from build123d import *

# Parameters (mm, degrees)
PLENUM_START          = -375
PLENUM_DEPTH          = 415
PLENUM_START_2        = -360
PLENUM_RIBS_DEPTH     = 385
RUNNER_START          = -6.1
RUNNER_1_DEPTH        = 36
RUNNER_START_2        = -29.9
RUNNER_2_DEPTH        = 36
RUNNER_START_3        = -117.86
RUNNER_3_DEPTH        = 36
RUNNER_START_4        = -141.66
RUNNER_4_DEPTH        = 36
RUNNER_START_5        = -229.62
RUNNER_5_DEPTH        = 36
RUNNER_START_6        = -253.42
RUNNER_6_DEPTH        = 36
RUNNER_START_7        = -341.38
RUNNER_7_DEPTH        = 36
RUNNER_START_8        = -365.18
RUNNER_8_DEPTH        = 36
THROTTLE_START        = 40
SKETCH11_R            = 44
THROTTLE_FLANGE_DEPTH = 8
THROTTLE_START_2      = 48
SKETCH12_R            = 36
THROTTLE_BODY_DEPTH   = 40
THROTTLE_START_3      = 50
SKETCH13_R            = 29
THROTTLE_BORE_DEPTH   = 40
FUEL_START            = -360
SKETCH14_R            = 8
FUEL_RAILS_DEPTH      = 390


with BuildPart() as part:
    # Sketch1 → Plenum (new body)
    with BuildSketch(Plane.XY.offset(PLENUM_START)):
        with BuildLine():
            Line((-50, 285), (50, 285))
            ThreePointArc((50, 285), (64.142135624, 290.857864376), (70, 305))
            Line((70, 305), (70, 335))
            ThreePointArc((70, 335), (64.142135624, 349.142135624), (50, 355))
            Line((50, 355), (-50, 355))
            ThreePointArc((-50, 355), (-64.142135624, 349.142135624), (-70, 335))
            Line((-70, 335), (-70, 305))
            ThreePointArc((-70, 305), (-64.142135624, 290.857864376), (-50, 285))
        make_face()
    extrude(amount=PLENUM_DEPTH)

    # Sketch2 → Plenum Ribs (add)
    with BuildSketch(Plane.XY.offset(PLENUM_START_2)):
        with BuildLine():
            Line((-50, 350), (-42, 350))
            Line((-42, 350), (-42, 359))
            ThreePointArc((-42, 359), (-42.878679656, 361.121320344), (-45, 362))
            Line((-45, 362), (-47, 362))
            ThreePointArc((-47, 362), (-49.121320344, 361.121320344), (-50, 359))
            Line((-50, 359), (-50, 350))
        make_face()
        with BuildLine():
            Line((-4, 350), (4, 350))
            Line((4, 350), (4, 359))
            ThreePointArc((4, 359), (3.121320344, 361.121320344), (1, 362))
            Line((1, 362), (-1, 362))
            ThreePointArc((-1, 362), (-3.121320344, 361.121320344), (-4, 359))
            Line((-4, 359), (-4, 350))
        make_face()
        with BuildLine():
            Line((42, 350), (50, 350))
            Line((50, 350), (50, 359))
            ThreePointArc((50, 359), (49.121320344, 361.121320344), (47, 362))
            Line((47, 362), (45, 362))
            ThreePointArc((45, 362), (42.878679656, 361.121320344), (42, 359))
            Line((42, 359), (42, 350))
        make_face()
    extrude(amount=PLENUM_RIBS_DEPTH)

    # Sketch3 → Runner 1 (add)
    with BuildSketch(Plane.XY.offset(RUNNER_START)):
        with BuildLine():
            Line((132.900719524, 234.724096015), (115.737566336, 251.887249203))
            ThreePointArc((115.737566336, 251.887249203), (114.502776925, 252.936394099), (113.114761283, 253.772350127))
            Line((113.114761283, 253.772350127), (28.879343102, 295.60957816))
            Line((28.879343102, 295.60957816), (51.120656898, 340.39042184))
            Line((51.120656898, 340.39042184), (142.684314275, 294.913475254))
            ThreePointArc((142.684314275, 294.913475254), (144.072329917, 294.077519226), (145.307119327, 293.02837433))
            Line((145.307119327, 293.02837433), (168.256058583, 270.079435074))
            Line((168.256058583, 270.079435074), (132.900719524, 234.724096015))
        make_face()
    extrude(amount=RUNNER_1_DEPTH)

    # Sketch4 → Runner 2 (add)
    with BuildSketch(Plane.XY.offset(RUNNER_START_2)):
        with BuildLine():
            Line((-168.256058583, 270.079435074), (-145.307119327, 293.02837433))
            ThreePointArc((-145.307119327, 293.02837433), (-144.072329917, 294.077519226), (-142.684314275, 294.913475254))
            Line((-142.684314275, 294.913475254), (-51.120656898, 340.39042184))
            Line((-51.120656898, 340.39042184), (-28.879343102, 295.60957816))
            Line((-28.879343102, 295.60957816), (-113.114761283, 253.772350127))
            ThreePointArc((-113.114761283, 253.772350127), (-114.502776925, 252.936394099), (-115.737566336, 251.887249203))
            Line((-115.737566336, 251.887249203), (-132.900719524, 234.724096015))
            Line((-132.900719524, 234.724096015), (-168.256058583, 270.079435074))
        make_face()
    extrude(amount=RUNNER_2_DEPTH)

    # Sketch5 → Runner 3 (add)
    with BuildSketch(Plane.XY.offset(RUNNER_START_3)):
        with BuildLine():
            Line((132.900719524, 234.724096015), (115.737566336, 251.887249203))
            ThreePointArc((115.737566336, 251.887249203), (114.502776925, 252.936394099), (113.114761283, 253.772350127))
            Line((113.114761283, 253.772350127), (28.879343102, 295.60957816))
            Line((28.879343102, 295.60957816), (51.120656898, 340.39042184))
            Line((51.120656898, 340.39042184), (142.684314275, 294.913475254))
            ThreePointArc((142.684314275, 294.913475254), (144.072329917, 294.077519226), (145.307119327, 293.02837433))
            Line((145.307119327, 293.02837433), (168.256058583, 270.079435074))
            Line((168.256058583, 270.079435074), (132.900719524, 234.724096015))
        make_face()
    extrude(amount=RUNNER_3_DEPTH)

    # Sketch6 → Runner 4 (add)
    with BuildSketch(Plane.XY.offset(RUNNER_START_4)):
        with BuildLine():
            Line((-168.256058583, 270.079435074), (-145.307119327, 293.02837433))
            ThreePointArc((-145.307119327, 293.02837433), (-144.072329917, 294.077519226), (-142.684314275, 294.913475254))
            Line((-142.684314275, 294.913475254), (-51.120656898, 340.39042184))
            Line((-51.120656898, 340.39042184), (-28.879343102, 295.60957816))
            Line((-28.879343102, 295.60957816), (-113.114761283, 253.772350127))
            ThreePointArc((-113.114761283, 253.772350127), (-114.502776925, 252.936394099), (-115.737566336, 251.887249203))
            Line((-115.737566336, 251.887249203), (-132.900719524, 234.724096015))
            Line((-132.900719524, 234.724096015), (-168.256058583, 270.079435074))
        make_face()
    extrude(amount=RUNNER_4_DEPTH)

    # Sketch7 → Runner 5 (add)
    with BuildSketch(Plane.XY.offset(RUNNER_START_5)):
        with BuildLine():
            Line((132.900719524, 234.724096015), (115.737566336, 251.887249203))
            ThreePointArc((115.737566336, 251.887249203), (114.502776925, 252.936394099), (113.114761283, 253.772350127))
            Line((113.114761283, 253.772350127), (28.879343102, 295.60957816))
            Line((28.879343102, 295.60957816), (51.120656898, 340.39042184))
            Line((51.120656898, 340.39042184), (142.684314275, 294.913475254))
            ThreePointArc((142.684314275, 294.913475254), (144.072329917, 294.077519226), (145.307119327, 293.02837433))
            Line((145.307119327, 293.02837433), (168.256058583, 270.079435074))
            Line((168.256058583, 270.079435074), (132.900719524, 234.724096015))
        make_face()
    extrude(amount=RUNNER_5_DEPTH)

    # Sketch8 → Runner 6 (add)
    with BuildSketch(Plane.XY.offset(RUNNER_START_6)):
        with BuildLine():
            Line((-168.256058583, 270.079435074), (-145.307119327, 293.02837433))
            ThreePointArc((-145.307119327, 293.02837433), (-144.072329917, 294.077519226), (-142.684314275, 294.913475254))
            Line((-142.684314275, 294.913475254), (-51.120656898, 340.39042184))
            Line((-51.120656898, 340.39042184), (-28.879343102, 295.60957816))
            Line((-28.879343102, 295.60957816), (-113.114761283, 253.772350127))
            ThreePointArc((-113.114761283, 253.772350127), (-114.502776925, 252.936394099), (-115.737566336, 251.887249203))
            Line((-115.737566336, 251.887249203), (-132.900719524, 234.724096015))
            Line((-132.900719524, 234.724096015), (-168.256058583, 270.079435074))
        make_face()
    extrude(amount=RUNNER_6_DEPTH)

    # Sketch9 → Runner 7 (add)
    with BuildSketch(Plane.XY.offset(RUNNER_START_7)):
        with BuildLine():
            Line((132.900719524, 234.724096015), (115.737566336, 251.887249203))
            ThreePointArc((115.737566336, 251.887249203), (114.502776925, 252.936394099), (113.114761283, 253.772350127))
            Line((113.114761283, 253.772350127), (28.879343102, 295.60957816))
            Line((28.879343102, 295.60957816), (51.120656898, 340.39042184))
            Line((51.120656898, 340.39042184), (142.684314275, 294.913475254))
            ThreePointArc((142.684314275, 294.913475254), (144.072329917, 294.077519226), (145.307119327, 293.02837433))
            Line((145.307119327, 293.02837433), (168.256058583, 270.079435074))
            Line((168.256058583, 270.079435074), (132.900719524, 234.724096015))
        make_face()
    extrude(amount=RUNNER_7_DEPTH)

    # Sketch10 → Runner 8 (add)
    with BuildSketch(Plane.XY.offset(RUNNER_START_8)):
        with BuildLine():
            Line((-168.256058583, 270.079435074), (-145.307119327, 293.02837433))
            ThreePointArc((-145.307119327, 293.02837433), (-144.072329917, 294.077519226), (-142.684314275, 294.913475254))
            Line((-142.684314275, 294.913475254), (-51.120656898, 340.39042184))
            Line((-51.120656898, 340.39042184), (-28.879343102, 295.60957816))
            Line((-28.879343102, 295.60957816), (-113.114761283, 253.772350127))
            ThreePointArc((-113.114761283, 253.772350127), (-114.502776925, 252.936394099), (-115.737566336, 251.887249203))
            Line((-115.737566336, 251.887249203), (-132.900719524, 234.724096015))
            Line((-132.900719524, 234.724096015), (-168.256058583, 270.079435074))
        make_face()
    extrude(amount=RUNNER_8_DEPTH)

    # Sketch11 → Throttle Flange (add)
    with BuildSketch(Plane.XY.offset(THROTTLE_START)):
        with Locations(Location((0, 320, 0), (0, 0, 127.301790292))):
            Circle(SKETCH11_R)
    extrude(amount=THROTTLE_FLANGE_DEPTH)

    # Sketch12 → Throttle Body (add)
    with BuildSketch(Plane.XY.offset(THROTTLE_START_2)):
        with Locations((0, 320)):
            Circle(SKETCH12_R)
    extrude(amount=THROTTLE_BODY_DEPTH)

    # Sketch13 → Throttle Bore (cut)
    with BuildSketch(Plane.XY.offset(THROTTLE_START_3)):
        with Locations((0, 320)):
            Circle(SKETCH13_R)
    extrude(amount=THROTTLE_BORE_DEPTH, mode=Mode.SUBTRACT)

    # Sketch14 → Fuel Rails (add)
    with BuildSketch(Plane.XY.offset(FUEL_START)):
        with Locations((106.963899649, 318.237487596)):
            Circle(SKETCH14_R)
        with Locations(Location((-106.963899649, 318.237487596, 0), (0, 0, 245.09441194))):
            Circle(SKETCH14_R)
    extrude(amount=FUEL_RAILS_DEPTH)


solid = part.part
Model file for the job. Use its own axes, mm. A direction names the side the tool comes from. Give positions to 0.01 mm unless a question says otherwise; leave off trailing zeros. Order: outer loops, then holes, each group sorted by start corner. A loop starts at its lowest first (then second) coordinate and runs counter-clockwise, first axis right, second up. Notation, with made-up numbers: (-33.5, 35.25) -> (-11.5, 35.25) arc R33 ccw to (-11.5, 65.25) -> close; hole circle Ø10 at (17, 27.5). An arc over 180 degrees is marked (long way). Use CSV: the item, a comma, the result in double quotes.
1. Drill centre lines: line 1 along Z through (x, y) = (-110, 306); line 2 along Z through (x, y) = (129.5, 251.5); line 3 along X through (y, z) = (318, -46.5). Where is each one in solid material? Low to high. Write a range as from..to.
Outcome:
line 1,"-365.18..-329.18, -253.42..-217.42, -141.66..-105.66, -29.9..6.1"
line 2,"-341.38..-305.38, -229.62..-193.62, -117.86..-81.86, -6.1..29.9"
line 3,"-114.96..-98.97, -70..70, 98.97..114.96"
2. Drop flat-ended pins along their axis: pin 1 (1 mm diameter, centred on x = 112.5, z = -291.5, fed in from -Y); pin 2 (3 mm diameter, centred on y = 273.5, z = -220, fed in from -X); pin 3 (5.5 mm diameter, centred on x = -46.5, y = 359, fed in from +Z); pin 4 (5.5 mm diameter, centred on x = -1, y = 357.5, fed in from -Z). Give the stop position or say it passes through.
Outcome:
pin 1,"y = 312.02"
pin 2,"x = -166.34"
pin 3,"z = 25"
pin 4,"z = -375"
3. Mould opens along Z. For faces 1 (the flat face through (-108, 284, -329.18)), 2 (the flat face through (2, 350, 88)), 3 (the cylindrical face through (-64.297, 291.014, -170.405)), 4 (the flat face through (-156.942, 281.393, -347.432)) say: +Z half, -Z half, draft (parallel to the pull), parting line (faces both ways), or undercut.
Outcome:
face 1,"undercut"
face 2,"+Z half"
face 3,"undercut"
face 4,"draft"
4. Band-saw the part on B-B, the plane z = -46. Give the cut face in (x, y), then the cut area to 3 significant figures.
Outcome:
outline,"circle Ø16 at (-106.96, 318.24); (-70, 305) arc R20 ccw to (-50, 285) -> (50, 285) arc R20 ccw to (70, 305) -> (70, 335) arc R20 ccw to (50, 355) -> (50, 359) arc R3 ccw to (47, 362) -> (45, 362) arc R3 ccw to (42, 359) -> (42, 355) -> (4, 355) -> (4, 359) arc R3 ccw to (1, 362) -> (-1, 362) arc R3 ccw to (-4, 359) -> (-4, 355) -> (-42, 355) -> (-42, 359) arc R3 ccw to (-45, 362) -> (-47, 362) arc R3 ccw to (-50, 359) -> (-50, 355) arc R20 ccw to (-70, 335) -> close; circle Ø16 at (106.96, 318.24)"
area,"10,000 mm²"
5. Band-saw the part on A-A, the plane y = 246. Count the separate pieces of the cut face and the enclosed holes in it, then the cut area to 3 significant figures.
Outcome:
separate pieces,"8"
enclosed holes,"0"
area,"6,490 mm²"
6. Band-saw the part on C-C, the plane x = -57.5. Give the cut face in (y, z), then the cut area to 3 significant figures.
Outcome:
outline,"(281.39, -365.18) -> (286.46, -365.18) -> (286.46, -375) -> (353.54, -375) -> (353.54, 40) -> (286.46, 40) -> (286.46, 6.1) -> (281.39, 6.1) -> (281.39, -29.9) -> (286.46, -29.9) -> (286.46, -105.66) -> (281.39, -105.66) -> (281.39, -141.66) -> (286.46, -141.66) -> (286.46, -217.42) -> (281.39, -217.42) -> (281.39, -253.42) -> (286.46, -253.42) -> (286.46, -329.18) -> (281.39, -329.18) -> close"
area,"28,600 mm²"
7. 3-axis set-ups, long thin cutter, end or side, ignore diameter. For faces 5 (the flat face through (82.116, 269.168, 11.648)), 6 (the flat face through (156.621, 281.715, 11.648)), 7 (the cylindrical face through (-7.804, 284.856, 67.72)): which of +Z, -Z, +X, -X, +Y, -Y reach the whole face in a straight line?
Outcome:
face 5,"+Z, -Z, -Y"
face 6,"+Z, -Z, +X, +Y"
face 7,"+Z"
